Build history of the part. All positions in model axes, mm. Face numbers are marked on the shaded views. A direction names the side the tool comes from. Give positions to 0.01 mm unless a question says otherwise; leave off trailing zeros. Loops run counter-clockwise (first coordinate to the right, second up) from the corner with the lowest first, then second, coordinate; pieces in that order, holes last. Notation, with made-up numbers: (53.25, 28) -> (79.25, 28) arc R26 ccw to (79.25, 49) -> close; hole circle Ø8 at (89.5, -20.75). An arc over 180 degrees is marked (long way). Answer as a JSON object with one key per item and string values. Group by question number.
Q1. Band-saw the part on A-A, the plane y = 77. Write the cut outline in (x, z), plus the area to 3 significant figures.
Q2. Band-saw the part on C-C, the plane x = 98. Write the cut outline in (y, z).
Q3. Band-saw the part on B-B, the plane z = 106. Write the cut outline in (x, y), plus the area to 3 significant figures.
Q4. Wall check: probe 1 along X at (y, z) = (36, 87); probe 2 along X at (y, z) = (120, 5); probe 3 along X at (y, z) = (4, 120). Give the ranges that are in metal, low to high. Write a range as from..to.
Q5. Band-saw the part on D-D, the plane x = 151. Write the cut outline in (y, z).
Q6. Drop flat-ended pins along their axis: pin 1 (7 mm diameter, centred on x = 167, z = 3.5, fed in from -Y); pin 2 (6 mm diameter, centred on x = 103, y = 60.5, fed in from +Z); pin 3 (12 mm diameter, centred on x = 64.5, z = 25, fed in from +Y). Give the stop position or say it passes through.
Q7. Tool access for the marked faces 1 and 2: list every direction of +Z, -Z, +X, -X, +Y, -Y with a clear straight run to the whole face (end or side of a thin tool).
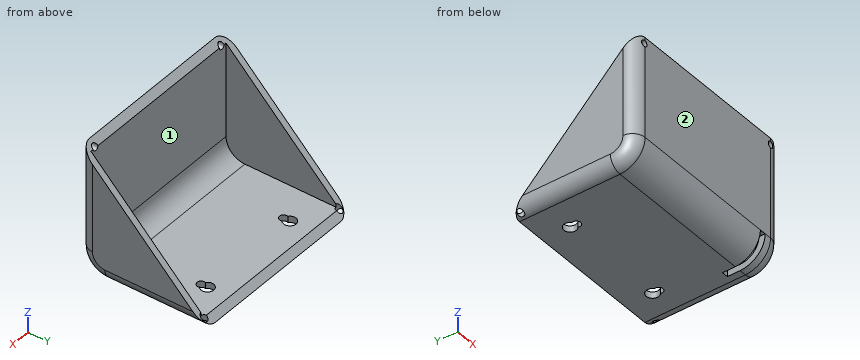
Autodesk Inventor part; units mm, degrees
ref_plane "YZ Plane" through (0, 0, 0) normal (1, 0, 0) x (0, 1, 0)
ref_plane "XZ Plane" through (0, 0, 0) normal (0, 1, 0) x (-1, 0, 0)
ref_plane "XY Plane" through (0, 0, 0) normal (0, 0, 1) x (1, 0, 0)
sketch "Sketch1" plane through (0, 0, 0) normal (1, 0, 0) x (0, 1, 0)
  line L0 (0, 0) -> (127, 0)
  line L1 (0, 0) -> (0, 127)
  line L2 (0, 127) -> (127, 0)
  dimension "d0" = 127
  dimension "d1" = 127
extrude "Extrusion1" add sketch "Sketch1" along normal blind 190.5
fillet "Fillet1" radius 25.4 1 edges at (95.25, 0, 0)
shell "Shell1" thickness 6.35 removed faces 1 at (127, 84.6667, 42.3333)
fillet "Fillet2" radius 12.7 6 edges at (190.5, 7.4395, 7.4395) (190.5, 0, 76.2) (190.5, 76.2, 0) (0, 7.4395, 7.4395) (0, 0, 76.2) (0, 76.2, 0)
sketch "Sketch2" plane through (177.8, 127, 0) normal (0, 0, -1) x (-1, 0, 0)
  line L0 (7.0063, -88.7561) -> (13.3563, -88.7561)
  line L1 (13.3563, -88.7561) -> (13.3563, -152.2561)
  line L2 (13.3563, -152.2561) -> (7.0063, -152.2561)
  line L3 (7.0063, -152.2561) -> (7.0063, -88.7561)
  point P0 (177.8, -127)
  dimension "d7" = 6.35
  dimension "d8" = 63.5
extrude "Extrusion2" cut sketch "Sketch2" against normal blind 25.4
sketch "Sketch3" plane through (177.8, 127, 0) normal (0, 0, -1) x (-1, 0, 0)
  circle A0 centre (26.2137, -27.9058) radius 6.35
  circle A1 centre (134.6629, -27.9058) radius 6.35
  point P0 (177.8, -127)
  dimension "d11" = 12.7
  dimension "d12" = 12.7
extrude "Extrusion3" cut sketch "Sketch3" against normal blind 25.4
sketch "Sketch4" plane through (177.8, 127, 0) normal (0, 0, -1) x (-1, 0, 0)
  circle A0 centre (26.2137, -27.9058) radius 6.35
  circle A1 centre (26.2137, -34.2558) radius 4.1275
  circle A2 centre (134.749, -34.2558) radius 4.1275
  point P0 (177.8, -127)
  dimension "d15" = 8.255
  dimension "d16" = 8.255
extrude "Extrusion4" cut sketch "Sketch4" against normal blind 25.4 contours A1 A0 | A0 A1 | A2 picked at (25.4127, -32.8707) picked at (27.1236, -35.5058)
sketch "Sketch5" plane through (177.8, 127, 0) normal (0, 0, -1) x (-1, 0, 0)
  point P0 (177.8, -127)
  point P1 (-6.35, -6.35)
  point P2 (171.45, -6.35)
  point P3 (171.45, -6.35)
hole "Hole1" at (184.15, 120.65, 0) at (6.35, 120.65, 0) direction (0, 0, 1) diameter 6.35 end through all
sketch "Sketch6" plane through (12.7, 0, 127) normal (0, -1, 0) x (1, 0, 0)
  line L0 (171.45, -6.35) -> (-6.35, -6.35)
  point P0 (-12.7, -127)
  point P1 (-0.7443, -6.35)
  point P2 (165.3424, -6.35)
hole "Hole2" at (11.9557, 0, 120.65) at (178.0424, 0, 120.65) direction (0, 1, 0) diameter 6.35 end through all
properties part number "shell"
Worked answers:
{
 "1": {"outline": "(0, 12.7) arc R12.7 ccw to (12.7, 0) -> (177.8, 0) arc R12.7 ccw to (190.5, 12.7) -> (190.5, 50) -> (184.15, 50) -> (184.15, 6.35) -> (6.35, 6.35) -> (6.35, 50) -> (0, 50) -> close", "area": "1,690 mm2"},
 "2": {"outline": "(0, 25.4) arc R25.4 ccw to (25.4, 0) -> (127, 0) -> (120.65, 6.35) -> (25.4, 6.35) arc R19.05 cw to (6.35, 25.4) -> (6.35, 120.65) -> (0, 127) -> close"},
 "3": {"outline": "(0, 12.7) arc R12.7 ccw to (12.7, 0) -> (177.8, 0) arc R12.7 ccw to (190.5, 12.7) -> (190.5, 21) -> (184.15, 21) -> (184.15, 6.35) -> (6.35, 6.35) -> (6.35, 21) -> (0, 21) -> close", "area": "1,330 mm2"},
 "4": {"probe 1": "0..6.35, 184.15..190.5", "probe 2": "2.6..3.24, 9.46..181.04, 187.26..187.9", "probe 3": "3.45..8.85, 15.06..174.93, 181.15..187.05"},
 "5": {"outline": "(0, 25.4) arc R25.4 ccw to (25.4, 0) -> (88.66, 0) -> (88.66, 6.35) -> (25.4, 6.35) arc R19.05 cw to (6.35, 25.4) -> (6.35, 120.65) -> (0, 127) -> close; (105.42, 0) -> (127, 0) -> (120.65, 6.35) -> (105.42, 6.35) -> close"},
 "6": {"pin 1": "y = 9.14", "pin 2": "z = 6.35", "pin 3": "y = 7.46"},
 "7": {"face 1": "+Z, +Y", "face 2": "+Z, -Z, +X, -X, -Y"}
}
